from build123d import *

# Parameters (mm, degrees)
BOSS_EXTRUDE1_DEPTH           = 127
BOSS_EXTRUDE1_DEPTH_BACK      = 127
SKETCH3_W                     = 31.75
SKETCH3_H                     = 31.75
SKETCH3_W_2                   = 25.4
SKETCH3_H_2                   = 25.4
F_10_CLEARANCE_HOLE1_D        = 4.9784
SKETCH7_R                     = 14.2875
CUT_EXTRUDE1_DEPTH            = 7.62
CUT_EXTRUDE2_START            = -7.62
SKETCH8_R                     = 14.2875
CUT_EXTRUDE2_DEPTH            = 7.62
F_10_CLEARANCE_HOLE2_D        = 4.9784
SKETCH12_R                    = 6.35
CUT_EXTRUDE3_DEPTH            = 132.867653824
TAP_DRILL_FOR_8_32_TAP1_D     = 3.4544
TAP_DRILL_FOR_8_32_TAP1_DEPTH = 5.08
TAP_DRILL_FOR_8_32_TAP1_TIP   = 1.037806461


with BuildPart() as part:
    # Sketch3 → Boss-Extrude1 (new, two sides: drawn at the far end of the back side and taken through both)
    with BuildSketch(Plane.XY.offset(-BOSS_EXTRUDE1_DEPTH_BACK)):
        Rectangle(SKETCH3_W, SKETCH3_H)
        Rectangle(SKETCH3_W_2, SKETCH3_H_2, mode=Mode.SUBTRACT)
    extrude(amount=BOSS_EXTRUDE1_DEPTH + BOSS_EXTRUDE1_DEPTH_BACK)

    # #10 Clearance Hole1 (through all)
    with Locations(Plane(origin=(0, 15.875, 0), x_dir=(1, 0, 0), z_dir=(0, 1, 0))):
        with Locations((-9.525, -117.475), (9.525, -117.475), (0, -98.247200001), (-7.111939052, -75.171256705)):
            Hole(F_10_CLEARANCE_HOLE1_D / 2)

    # Sketch7 → Cut-Extrude1 (cut)
    with BuildSketch(Plane(origin=(0, 15.875, 0), x_dir=(1, 0, 0), z_dir=(0, 1, 0))):
        with Locations(Location((0, 17.8816, 0), (0, 0, 270))):
            Circle(SKETCH7_R)
    extrude(amount=-CUT_EXTRUDE1_DEPTH, mode=Mode.SUBTRACT)

    # Sketch8 → Cut-Extrude2 (cut)
    with BuildSketch(Plane.XZ.offset(15.875).offset(CUT_EXTRUDE2_START)):
        with Locations(Location((0, -17.8816, 0), (0, 0, 90))):
            Circle(SKETCH8_R)
    extrude(amount=CUT_EXTRUDE2_DEPTH, mode=Mode.SUBTRACT)

    # #10 Clearance Hole2 (through all)
    with Locations(Plane(origin=(15.875, 0, 0), x_dir=(0, 0, -1), z_dir=(1, 0, 0))):
        with Locations((-82.55, -3.175), (114.3, -3.175), (40.132, -3.175)):
            Hole(F_10_CLEARANCE_HOLE2_D / 2)

    # Sketch12 → Cut-Extrude3 (cut, through all)
    with BuildSketch(Plane(origin=(0, 15.875, 0), x_dir=(1, 0, 0), z_dir=(0, 1, 0))):
        with Locations((-20.955, -94.557636183)):
            Circle(SKETCH12_R)
    extrude(amount=-CUT_EXTRUDE3_DEPTH, mode=Mode.SUBTRACT)

    # Tap Drill for #8-32 Tap1
    with Locations(Plane(origin=(0, -15.875, 0), x_dir=(-1, 0, 0), z_dir=(0, -1, 0))):
        with Locations((0, 35.9156), (0, -0.1524)):
            Hole(TAP_DRILL_FOR_8_32_TAP1_D / 2, depth=TAP_DRILL_FOR_8_32_TAP1_DEPTH)
            with Locations((0, 0, -(TAP_DRILL_FOR_8_32_TAP1_DEPTH + TAP_DRILL_FOR_8_32_TAP1_TIP / 2))):  # 118° drill point
                Cone(0, TAP_DRILL_FOR_8_32_TAP1_D / 2, TAP_DRILL_FOR_8_32_TAP1_TIP, mode=Mode.SUBTRACT)


solid = part.part
Verification items for the finished model (mm, model axes). A direction names the side the tool comes from. Coordinates: 2 decimals unless noted, no trailing zeros. Order: outer loops, then holes, each group sorted by start corner. A loop starts at its lowest first (then second) coordinate and runs counter-clockwise, first axis right, second up.
1. Sectioned sample at D-D, the plane x = 9.5. Record the cut outline in (y, z) (3 decimals), and give its area (3 significant figures).
Results found:
outline: (-15.875, -127) - (-12.7, -127) - (-12.7, -28.553) - (-15.875, -28.553) - close; (-15.875, -7.21) - (-12.7, -7.21) - (-12.7, 114.986) - (-15.875, 114.986) - close; (-15.875, 119.964) - (-12.7, 119.964) - (-12.7, 127) - (-15.875, 127) - close; (12.7, -127) - (15.875, -127) - (15.875, -28.553) - (12.7, -28.553) - close; (12.7, -7.21) - (15.875, -7.21) - (15.875, 114.986) - (12.7, 114.986) - close; (12.7, 119.964) - (15.875, 119.964) - (15.875, 127) - (12.7, 127) - close
area: 1,450 mm2
2. Sectioned sample at A-A, the plane z = -114.3. Record the cut outline in (x, y) (3 decimals), and give its area (3 significant figures).
Results found:
outline: (-15.875, -15.875) - (15.875, -15.875) - (15.875, -5.664) - (12.7, -5.664) - (12.7, -12.7) - (-12.7, -12.7) - (-12.7, -5.664) - (-15.875, -5.664) - close; (-15.875, -0.686) - (-12.7, -0.686) - (-12.7, 12.7) - (12.7, 12.7) - (12.7, -0.686) - (15.875, -0.686) - (15.875, 15.875) - (-15.875, 15.875) - close
area: 331 mm2
3. Scan lines: line 1 (Z direction, x = 0, y = 14); line 2 (Y direction, x = 11, z = 79) (3 decimals); line 3 (Z direction, x = -10, y = 13). Record each from-to range of solid material in increasing order.
Results found:
line 1: z = -127 to -32.17, -3.59 to 95.76, 100.74 to 127
line 2: y = -15.875 to -12.7, 12.7 to 15.875
line 3: z = -127 to -28.09, -7.68 to 115.03, 119.92 to 127
4. Release check for a two-part mould opening along X. For faces 4 (the face through (14.27, -3.07, -42.62)), 5 (the face through (0, -12.7, 57)), 6 (the face through (-15.875, 0, -20)) record: +X half, -X half, draft (parallel to the pull), parting line (faces both ways), or undercut.
Results found:
face 4: draft
face 5: undercut
face 6: -X half
5. Set-up check for faces 1 (the face through (-12.7, 0, -2)), 2 (the face through (-14.605, 0.222, 94.615)), 3 (the face through (0.628, 13.812, -32.155)): record each of +Z, -Z, +X, -X, +Y, -Y from which the full face is reachable in a straight line by a thin tool's end or side.
Results found:
face 1: +Z, -Z
face 2: -X, +Y, -Y
face 3: +Y
6. Go/stop test with flat-tipped pins: pin 1 Ø8 at (x, z) = (-7.11, 75.17) entering from +Y (3 decimals); pin 2 Ø3 at (x, z) = (0, -35.92) entering from -Y; pin 3 Ø0.8 at (x, z) = (-13.5, -21) entering from +Y (3 decimals); pin 4 Ø0.8 at (x, z) = (-13, -20) entering from -Y (3 decimals). Record where each tip stops, or that it passes through.
Results found:
pin 1: stops at y = 15.875
pin 2: stops at y = 12.7
pin 3: stops at y = 8.255
pin 4: stops at y = -8.255
7. Sectioned sample at B-B, the plane y = 3.5. Record the cut outline in (x, z) (3 decimals), and give its area (3 significant figures).
Results found:
outline: (-15.875, -127) - (-12.7, -127) - (-12.7, 127) - (-15.875, 127) - (-15.875, 98.368) arc R6.35 cw to (-15.875, 90.748) - close; (12.7, -127) - (15.875, -127) - (15.875, 127) - (12.7, 127) - close
area: 1,610 mm2
8. Sectioned sample at C-C, the plane z = 41. Record the cut outline in (x, y) (3 decimals).
Results found:
outline: (-15.875, -15.875) - (15.875, -15.875) - (15.875, 15.875) - (-15.875, 15.875) - close; hole (-12.7, -12.7) - (12.7, -12.7) - (12.7, 12.7) - (-12.7, 12.7) - close
